from build123d import *

# Parameters (mm, degrees)
SKETCH_R  = 4.3
PAD_DEPTH = 8


with BuildPart() as part:
    # Sketch → Pad (new body)
    with BuildSketch(Plane.XY):
        with BuildLine():
            Line((20, 0), (50, 0))
            ThreePointArc((50, 0), (67.201528, 4.717883), (79.589256, 17.551244))
            Line((79.589256, 17.551244), (235, 302))
            Line((235, 302), (285, 302))
            Line((285, 302), (440.410744, 17.551244))
            ThreePointArc((440.410744, 17.551244), (452.798472, 4.717883), (470, 0))
            Line((470, 0), (500, 0))
            ThreePointArc((500, 0), (510.203305, 5.811034), (510.410744, 17.551244))
            Line((510.410744, 17.551244), (364.589256, 284.448756))
            ThreePointArc((350.956802, 321.58705), (356.39416, 302.511758), (364.589256, 284.448756))
            Line((350.956802, 321.58705), (315.053998, 495.516187))
            ThreePointArc((315.053998, 495.516187), (304.382337, 513.104291), (285, 520))
            Line((235, 520), (285, 520))
            ThreePointArc((235, 520), (215.617663, 513.104291), (204.946002, 495.516187))
            Line((204.946002, 495.516187), (169.043198, 321.58705))
            ThreePointArc((155.410744, 284.448756), (163.60584, 302.511758), (169.043198, 321.58705))
            Line((155.410744, 284.448756), (9.589256, 17.551244))
            ThreePointArc((9.589256, 17.551244), (9.796695, 5.811034), (20, 0))
        make_face()
        with Locations((245, 328)):
            Circle(SKETCH_R, mode=Mode.SUBTRACT)
        with Locations((275, 328)):
            Circle(SKETCH_R, mode=Mode.SUBTRACT)
        with Locations((275, 309)):
            Circle(SKETCH_R, mode=Mode.SUBTRACT)
        with Locations((245, 309)):
            Circle(SKETCH_R, mode=Mode.SUBTRACT)
        with Locations((490, 25)):
            Circle(SKETCH_R, mode=Mode.SUBTRACT)
        with Locations((450, 25)):
            Circle(SKETCH_R, mode=Mode.SUBTRACT)
        with Locations((70, 25)):
            Circle(SKETCH_R, mode=Mode.SUBTRACT)
        with Locations((30, 25)):
            Circle(SKETCH_R, mode=Mode.SUBTRACT)
        with Locations((225, 495)):
            Circle(SKETCH_R, mode=Mode.SUBTRACT)
        with Locations((295, 495)):
            Circle(SKETCH_R, mode=Mode.SUBTRACT)
    extrude(amount=PAD_DEPTH)


solid = part.part
Design review of the part built by this model. Coordinates are the model's own, in mm. A direction names the side the tool comes from. Give positions to 0.01 mm unless a question says otherwise; leave off trailing zeros. Loops run counter-clockwise (first coordinate to the right, second up) from the corner with the lowest first, then second, coordinate; pieces in that order, holes last. Notation, with made-up numbers: M 66,18.25 L 122,18.25 A19 cw 122,49.25 Z; hole C -19,72.5 d4. An arc over 180 degrees is marked long. Write item = value, one per line.
Q1. We need section D-D (y = 416). Give the boundary of the cut face in (x, z), plus the area to 3 significant figures.
Output values:
outline = M 188.53,0 L 331.47,0 L 331.47,8 L 188.53,8 Z
area = 1,140 mm^2
Q2. To check wall thickness, follow line 1 (Y direction, x = 274, z = 7.25); line 2 (Y direction, x = 245, z = 5.25); line 3 (X direction, y = 495, z = 4.75). State the ranges of each line that lie inside material, in increasing order. Write a range as [from, to].
Output values:
line_1 = [302, 304.82], [313.18, 323.82], [332.18, 520]
line_2 = [302, 304.7], [313.3, 323.7], [332.3, 520]
line_3 = [204.84, 220.7], [229.3, 290.7], [299.3, 315.16]
Q3. Draft analysis for pull direction X (two halves, no side actions). For faces 1 (the cylindrical face through (452.58, 4.85, 3.94)), 2 (the cylindrical face through (356.3, 302.77, 3.94)), 3 (the cylindrical face through (9.71, 5.96, 3.94)), 4 (the cylindrical face through (67, 4.6, 3.9)), state which applies: +X half, -X half, draft (parallel to the pull), parting line (faces both ways), or undercut.
Output values:
face_1 = undercut
face_2 = +X half
face_3 = -X half
face_4 = undercut
Q4. For faces 5 (the flat face through (156.207, 157.784, 3.944)), 6 (the flat face through (315, 261, 0)), list the 3-axis set-ups (+Z, -Z, +X, -X, +Y, -Y) from which the entire face can be reached by the end or side of a thin tool; tool diameter is ignored.
Output values:
face_5 = +Z, -Z, -Y
face_6 = -Z, +X, -X, +Y, -Y
Q5. We need section A-A (z = 1.75). Count the separate pieces of the cut face and the enclosed holes in it, plus the area to 3 significant figures.
Output values:
separate_pieces = 1
enclosed_holes = 10
area = 72,800 mm^2
Q6. We need section B-B (y = 46.5). Give the boundary of the cut face in (x, z).
Output values:
outline = M 25.41,0 L 95.41,0 L 95.41,8 L 25.41,8 Z; M 424.59,0 L 494.59,0 L 494.59,8 L 424.59,8 Z
Q7. We need section C-C (x = 416). Give the boundary of the cut face in (y, z), plus the area to 3 significant figures.
Output values:
outline = M 62.23,0 L 190.35,0 L 190.35,8 L 62.23,8 Z
area = 1,020 mm^2
Q8. Insertion check: pin 1 (3 mm diameter, centred on y = 154, z = 5, fed in from +X); pin 2 (10 mm diameter, centred on x = 295, y = 495, fed in from -Z); pin 3 (4 mm diameter, centred on x = 261, z = 5.5, fed in from -Y); pin 4 (3 mm diameter, centred on y = 252, z = 5.5, fed in from -X). Each pin has a flat end and moves straight along its axis. Give the tip position at first contact, or say it passes through.
Output values:
pin_1 = 436.68
pin_2 = 0
pin_3 = 302
pin_4 = 136.86
